Part print with two shaded views. Sizes in mm from the minimum x, y, z corner. Coordinates: 2 decimals unless noted, no trailing zeros. Write each loop counter-clockwise with the first axis right and the second up, starting at its lowest first coordinate (ties: lowest second). Pieces come first, ordered by that corner, then holes. Notation, with made-up numbers: (55.25, -11.75) - (74.25, -11.75) arc R25 ccw to (74.25, 7.25) - close; hole circle Ø8 at (33.25, -36.75). An arc over 180 degrees is marked (long way). Answer in a Markdown table with one row per item. Add a question column.
Q1. Pin check, flat tips, straight feed: pin 1 (1 mm diameter, centred on y = 0.5, z = 6, fed in from -X); pin 2 (0.6 mm diameter, centred on y = 1, z = 39.5, fed in from -X). Stop position of each tip, or through.
Q2. Band-saw the part on D-D (z = 15.5). List the corners of the cut face in (x, y).
Q3. Band-saw the part on C-C (y = 1.15). State how many separate pieces and enclosed holes the cut face has, and give its area (3 significant figures).
Q4. Band-saw the part on A-A (x = 46.5). List the corners of the cut face in (y, z).
Q5. Drill centre lines: line 1 along X through (y, z) = (1.05, 39); line 2 along X through (y, z) = (1.1, 20.5); line 3 along X through (y, z) = (1.75, 21). Where is each one in solid material? Low to high. Write a range as from..to.
Q6. Band-saw the part on B-B (x = 9). List the corners of the cut face in (y, z), and give its area (3 significant figures).
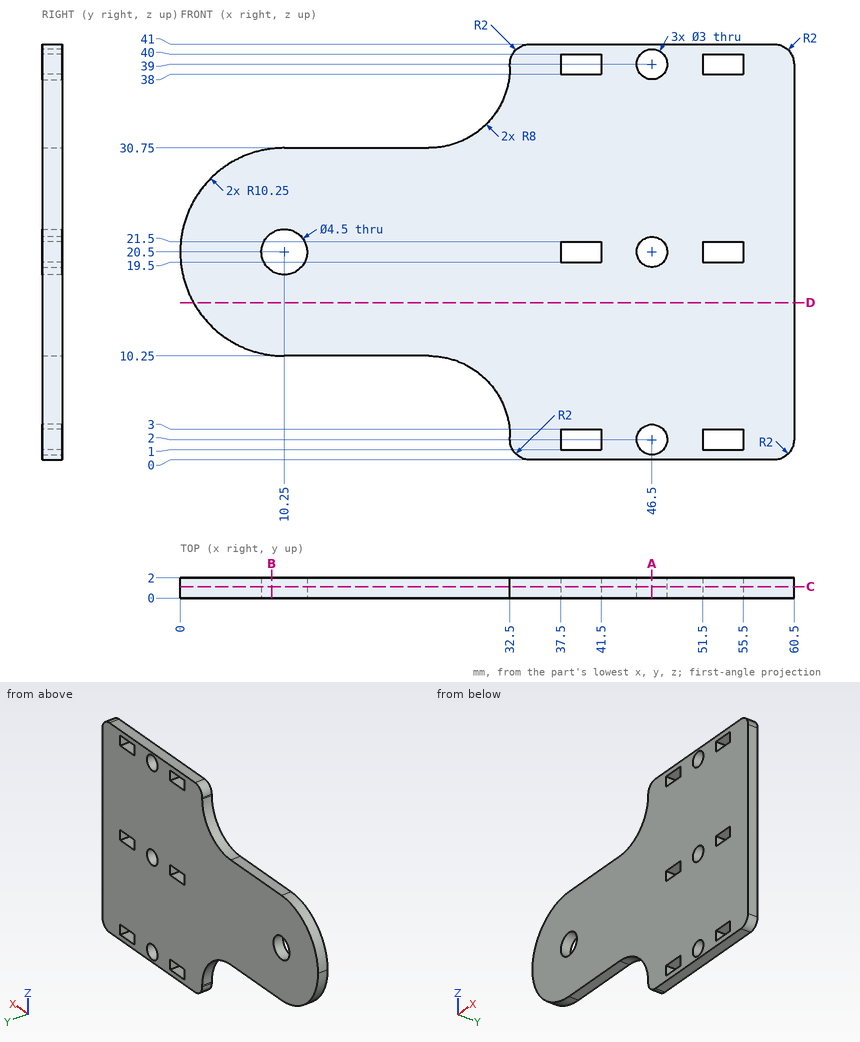
Checked values:
| question | item | result |
|---|---|---|
| 1 | pin 1 | stops at x = 31.28 |
| 1 | pin 2 | stops at x = 32.51 |
| 2 | outline | (1.3, 0) - (60.5, 0) - (60.5, 2) - (1.3, 2) - close |
| 3 | separate pieces | 1 |
| 3 | enclosed holes | 10 |
| 3 | area | 1,710 mm² |
| 4 | outline | (0, 0) - (2, 0) - (2, 0.5) - (0, 0.5) - close; (0, 3.5) - (2, 3.5) - (2, 19) - (0, 19) - close; (0, 22) - (2, 22) - (2, 37.5) - (0, 37.5) - close; (0, 40.5) - (2, 40.5) - (2, 41) - (0, 41) - close |
| 5 | line 1 | x = 32.5..37.5, 41.5..45, 48..51.5, 55.5..60.5 |
| 5 | line 2 | x = 0..8, 12.5..37.5, 41.5..45, 48..51.5, 55.5..60.5 |
| 5 | line 3 | x = 0.01..8.06, 12.44..37.5, 41.5..45.09, 47.91..51.5, 55.5..60.5 |
| 6 | outline | (0, 10.33) - (2, 10.33) - (2, 18.63) - (0, 18.63) - close; (0, 22.37) - (2, 22.37) - (2, 30.67) - (0, 30.67) - close |
| 6 | area | 33.2 mm² |
